Verification items for this drawing (mm, ordinates from the low corner). Round coordinates to 2 decimals unless told otherwise and drop trailing zeros. Loops run counter-clockwise (first coordinate to the right, second up) from the corner with the lowest first, then second, coordinate; pieces in that order, holes last. Notation, with made-up numbers: M 64,65 L 99,65 A24 cw 99,98 Z; hole C -32,-18.75 d9. An arc over 180 degrees is marked long. Use one line per item in the form item = value. Start each with the question number.
1. Material ranges on line 1 (Y direction, x = 342.9, z = 20) (3 decimals); line 2 (Y direction, x = 36, z = 16.75); line 3 (X direction, y = 221.5, z = 16.5), recorded low to high.
2. Cross-section at D-D (x = 224). Record the boundary of the cut face in (y, z), then the cut area to 3 significant figures.
3. Cross-section at A-A (z = 8.75). Record the boundary of the cut face in (x, y) (3 decimals).
4. Draft check along Y on the marked faces 1 and 2. Enter one of: pulls with the +Y half, pulls with the -Y half, needs draft (parallel to the pull), parting line crosses it, or undercut.
5. Go/stop test with a flat-tipped pin: pin 1 (10 mm diameter, centred on y = 190, z = 20.5, fed in from -X). Record where the tip stops, or that it passes through.
6. Cross-section at B-B (y = 342.9). Record the boundary of the cut face in (x, z) (3 decimals), then the cut area to 3 significant figures.
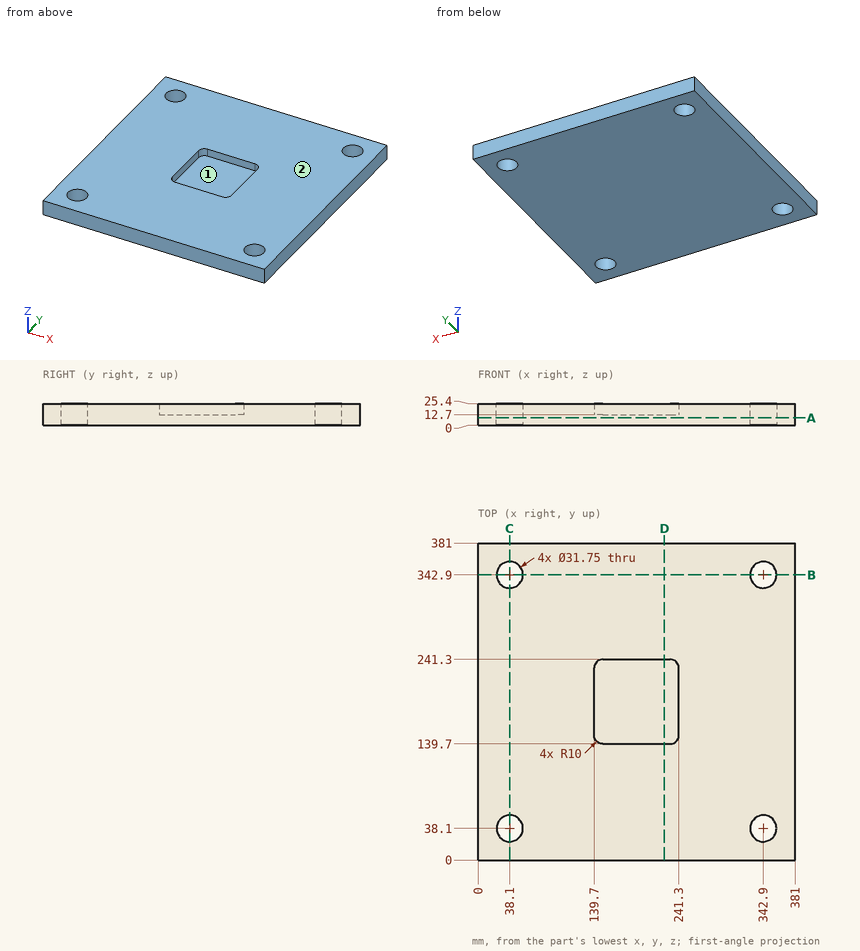
Reported:
q1.line_1 = 0 to 22.225, 53.975 to 327.025, 358.775 to 381
q1.line_2 = 0 to 22.36, 53.84 to 327.16, 358.64 to 381
q1.line_3 = 0 to 139.7, 241.3 to 381
q2.outline = M 0,0 L 381,0 L 381,25.4 L 241.3,25.4 L 241.3,12.7 L 139.7,12.7 L 139.7,25.4 L 0,25.4 Z
q2.area = 8,390 mm²
q3.outline = M 0,0 L 381,0 L 381,381 L 0,381 Z; hole C 38.1,38.1 d31.75; hole C 38.1,342.9 d31.75; hole C 342.9,38.1 d31.75; hole C 342.9,342.9 d31.75
q4.face_1 = undercut
q4.face_2 = needs draft
q5.pin_1 = 0
q6.outline = M 0,0 L 22.225,0 L 22.225,25.4 L 0,25.4 Z; M 53.975,0 L 327.025,0 L 327.025,25.4 L 53.975,25.4 Z; M 358.775,0 L 381,0 L 381,25.4 L 358.775,25.4 Z
q6.area = 8,060 mm²
